Build history of the part. All positions in model axes, mm. A direction names the side the tool comes from. Give positions to 0.01 mm unless a question says otherwise; leave off trailing zeros. Order: outer loops, then holes, each group sorted by start corner. A loop starts at its lowest first (then second) coordinate and runs counter-clockwise, first axis right, second up. Notation, with made-up numbers: (15, 21.5) - (72, 21.5) arc R18 ccw to (72, 39.5) - close; hole circle Ø7 at (88.25, 44). An arc over 180 degrees is marked (long way). Use a Markdown table: item, result.
Autodesk Inventor part; units mm, degrees
ref_plane "YZ Plane" through (0, 0, 0) normal (1, 0, 0) x (0, 1, 0)
ref_plane "XZ Plane" through (0, 0, 0) normal (0, 1, 0) x (-1, 0, 0)
ref_plane "XY Plane" through (0, 0, 0) normal (0, 0, 1) x (1, 0, 0)
sketch "Sketch1" plane through (0, 0, 0) normal (0, 1, 0) x (-1, 0, 0)
  circle A0 centre (0, -17.2028) radius 2.54
  circle A1 centre (0.1552, -22.2805) radius 2.54
  line L0 (0, -17.2028) -> (4.826, -17.2028) construction
  circle A2 centre (4.475, -19.6072) radius 2.54
  circle A3 centre (1.5434, -19.6969) radius 2.54
  circle A4 centre (1.5434, -19.6969) radius 6.35
  line L1 (0.1552, -22.2805) -> (0, -17.2028)
  line L2 (4.475, -19.6072) -> (0, -17.2028)
  line L3 (4.475, -19.6072) -> (0.1552, -22.2805)
  line L4 (2.3151, -20.9439) -> (0, -17.2028)
  line L5 (0.1552, -22.2805) -> (2.2375, -18.405)
  line L6 (0.0776, -19.7417) -> (4.475, -19.6072)
  point P0 (3.0726, -21.725)
  point P1 (2.6762, -21.9703)
  point P2 (-0.9776, -20.0071)
  point P3 (-0.9918, -19.5412)
  point P4 (2.5352, -17.3585)
  point P5 (2.9458, -17.5791)
  dimension "d3" = 5.08
  dimension "d7" = 5.08
  dimension "d8" = 12.7
  dimension "d14" = 5.08
  dimension "d15" = 5.08
extrude "Extrusion1" add sketch "Sketch1" along normal blind 4.7625 contours A0 A3 L2 L1 | L1 L4 A3 | A3 L1 L3 A1 | A2 A3 L3 L2 | A3 L4 L2 | A3 L5 L1 | L2 L6 A3 | A3 L3 L5 | L6 L3 A3 | A4
extrude "Extrusion2" add sketch "Sketch1" along normal blind 9.525
fillet "Fillet1" radius 3.175 1 edges at (4.8066, 9.525, -19.6969)
properties part number "PluckTool"
1) Wall check: line 1 (X direction, y = 1, z = -19.75); line 2 (Z direction, x = 1.5, y = 6); line 3 (Z direction, x = -3, y = 9). Give the ranges that are in metal, low to high. Write a range as from..to.
Computed:
| item | result |
|---|---|
| line 1 | x = -7.89..-4.08, 1..4.81 |
| line 2 | z = -25.27..-24.21, -20.35..-19.25, -15.15..-14.12 |
| line 3 | z = -24.4..-21.78, -17.54..-14.99 |
2) Slice it at B-B (y = 3). Write the cut outline in (x, z).
Computed:
| item | result |
|---|---|
| outline | circle Ø12.7 at (-1.54, -19.7); hole circle Ø5.08 at (-1.54, -19.7) |
3) Two-plate mould, pull along Z, no slides. Class faces 3 (the cylindrical face through (1.402, 7.11, -15.085)), 4 (the flat face through (-1.5, 0, -22.4)), 5 (the cylindrical face through (-0.167, 3.131, -13.498)), 6 (the cylindrical face through (-1.213, 3.637, -22.215)): +Z half, -Z half, draft (parallel to the pull), parting line (faces both ways), or undercut.
Computed:
| item | result |
|---|---|
| face 3 | undercut |
| face 4 | draft |
| face 5 | parting line |
| face 6 | undercut |
4) Tool access for faces 1 (the flat face through (-3, 9.525, -22)), 2 (the cylindrical face through (-7.01, 7.11, -19.45)): list every direction of +Z, -Z, +X, -X, +Y, -Y with a clear straight run to the whole face (end or side of a thin tool).
Computed:
| item | result |
|---|---|
| face 1 | +Z, -Z, +X, -X, +Y |
| face 2 | +Y |
5) Pin check, flat tips, straight feed: P1, Ø1.5, axis at x = -5.5, y = 7, coming from the -Z side; P2, Ø6, axis at x = -4.47, z = -19.61, coming from the +Y side (3 decimals); P3, Ø3, axis at x = -1.54, z = -19.7, coming from the -Y side; P4, Ø2, axis at y = 7.5, z = -20.5, coming from the -X side. Stop position of each tip, or through.
Computed:
| item | result |
|---|---|
| P1 | stops at z = -25.12 |
| P2 | stops at y = 9.525 |
| P3 | passes through |
| P4 | stops at x = -7.87 |
